The drawing under review shows one solid part. Ordinate dimensions are in mm from its lowest x, y, z. A direction names the side the tool comes from. Round coordinates to 2 decimals unless told otherwise and drop trailing zeros. Order: outer loops, then holes, each group sorted by start corner. A loop starts at its lowest first (then second) coordinate and runs counter-clockwise, first axis right, second up. Notation, with made-up numbers: M -6,3.25 L 45,3.25 A11 cw 45,16.25 Z; hole C -2.75,-34.5 d11. An arc over 180 degrees is marked long. Answer as a JSON object with one key per item and string values. Group by question number.
1. Add section C-C on x = 36.75. State the section outline as (y, z) points, and give its area (3 significant figures).
2. Add section A-A on z = 15. State the section outline as (x, y) points.
3. Machinability: for the marked faces 1, 2 and 3, which of the approach directions +Z, -Z, +X, -X, +Y, -Y give a long, thin tool a straight path to every point of the face, cutting with its end or side? Answer none if there is none.
4. To check wall thickness, follow probe 1 along X at (y, z) = (28.05, 15); probe 2 along Z at (x, y) = (51, 27); probe 3 along Y at (x, z) = (47.5, 18). State the ranges of each line that lie inside material, in increasing order. Write a range as [from, to].
5. Clearance check with flat-ended pins moving along their axes: P1, Ø4, axis at x = 31, z = 12, coming from the +Y side; P2, Ø3, axis at x = 3.75, z = 5, coming from the -Y side; P3, Ø1.5, axis at y = 15, z = 10.5, coming from the -X side; P4, Ø10, axis at y = 39, z = 11.5, coming from the +X side. State where each tip first meets the part, or that it passes through.
6. Add section D-D on y = 17.5. State the section outline as (x, z) points, and give its area (3 significant figures).
7. Add section B-B on x = 51.75. State the section outline as (y, z) points, and give its area (3 significant figures).
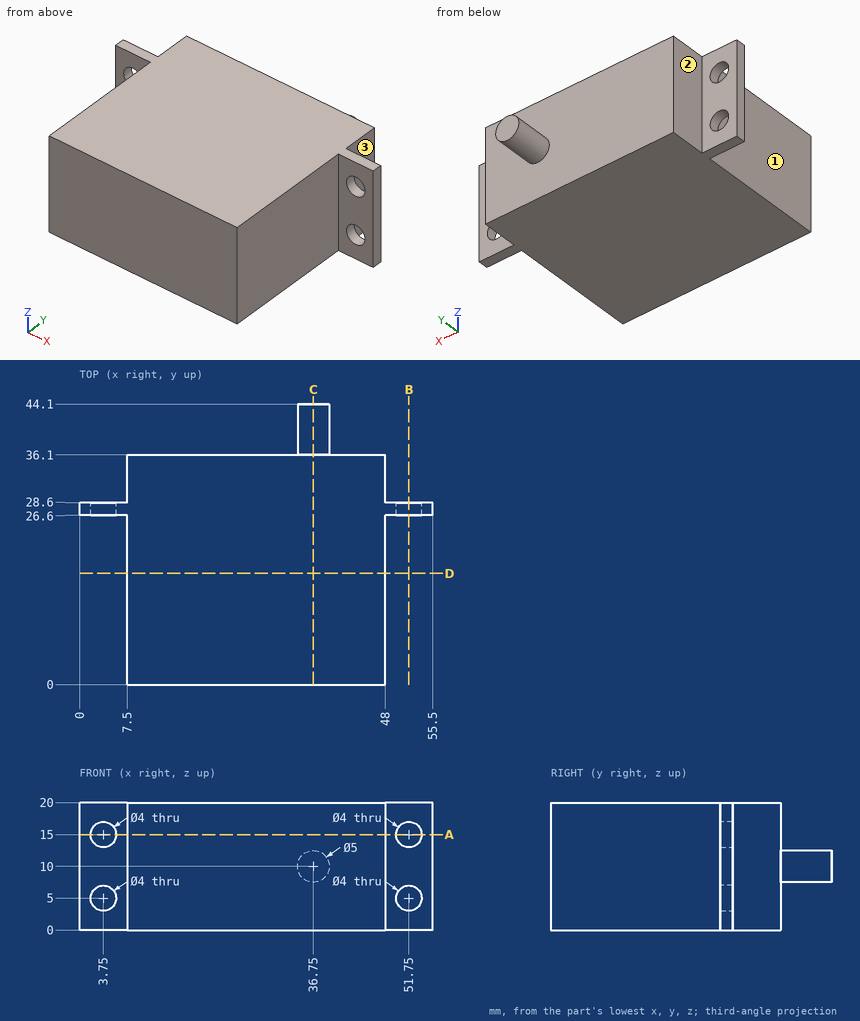
Recorded:
{
 "1": {"outline": "M 0,0 L 36.1,0 L 36.1,7.5 L 44.1,7.5 L 44.1,12.5 L 36.1,12.5 L 36.1,20 L 0,20 Z", "area": "762 mm²"},
 "2": {"outline": "M 0,26.6 L 1.75,26.6 L 1.75,28.6 L 0,28.6 Z; M 5.75,26.6 L 7.5,26.6 L 7.5,0 L 48,0 L 48,26.6 L 49.75,26.6 L 49.75,28.6 L 48,28.6 L 48,36.1 L 7.5,36.1 L 7.5,28.6 L 5.75,28.6 Z; M 53.75,26.6 L 55.5,26.6 L 55.5,28.6 L 53.75,28.6 Z"},
 "3": {"face 1": "+Z, -Z, -X, -Y", "face 2": "+Z, -Z, -X, +Y", "face 3": "+Z, -Z, +X, +Y"},
 "4": {"probe 1": "x = [0, 1.75], [5.75, 49.75], [53.75, 55.5]", "probe 2": "z = [0, 3.15], [6.85, 13.15], [16.85, 20]", "probe 3": "y = [0, 36.1]"},
 "5": {"P1": "stops at y = 36.1", "P2": "passes through", "P3": "stops at x = 7.5", "P4": "stops at x = 48"},
 "6": {"outline": "M 7.5,0 L 48,0 L 48,20 L 7.5,20 Z", "area": "810 mm²"},
 "7": {"outline": "M 26.6,0 L 28.6,0 L 28.6,3 L 26.6,3 Z; M 26.6,7 L 28.6,7 L 28.6,13 L 26.6,13 Z; M 26.6,17 L 28.6,17 L 28.6,20 L 26.6,20 Z", "area": "24.0 mm²"}
}
